```python
from build123d import *

# Parameters (mm, degrees)
SKETCH012_W     = 18.8
SKETCH012_H     = 47
PAD008_DEPTH    = 69
SKETCH036_W     = 14.1
SKETCH036_H     = 47
PAD016_DEPTH    = 2
SKETCH054_R     = 8
POCKET021_DEPTH = 18.801
SKETCH055_R     = 11
POCKET022_DEPTH = 7
CHAMFER001_SIZE = 12
SKETCH073_R     = 1.5
POCKET028_DEPTH = 19.2
FILLET003_R     = 3


with BuildPart() as part:
    # Sketch012 (on Face1 of ReferencePad001) → Pad008 (new body)
    with BuildSketch(Plane.XY.offset(18.8)):
        with Locations((-65.6, 0)):
            Rectangle(SKETCH012_W, SKETCH012_H)
    extrude(amount=PAD008_DEPTH)

    # Sketch036 (on Face5 of Pad008) → Pad016 (join)
    with BuildSketch(Plane(origin=(0, 0, 18.8), x_dir=(1, 0, 0), z_dir=(0, 0, -1))):
        with Locations((-67.95, 0)):
            Rectangle(SKETCH036_W, SKETCH036_H)
    extrude(amount=PAD016_DEPTH)

    # Sketch054 (on Face5 of Pad016) → Pocket021 (cut, through all)
    with BuildSketch(Plane(origin=(-75, 0, 18.8), x_dir=(0, -1, 0), z_dir=(-1, 0, 0))):
        with Locations((0, 56.2)):
            Circle(SKETCH054_R)
    extrude(amount=-POCKET021_DEPTH, mode=Mode.SUBTRACT)

    # Sketch055 (on Face5 of Pocket021) → Pocket022 (cut)
    with BuildSketch(Plane(origin=(-75, 0, 18.8), x_dir=(0, -1, 0), z_dir=(-1, 0, 0))):
        with Locations((0, 56.2)):
            Circle(SKETCH055_R)
    extrude(amount=-POCKET022_DEPTH, mode=Mode.SUBTRACT)

    # Chamfer001
    chamfer001_edges = [part.edges().sort_by_distance(p)[0] for p in [
        (-65.6, -23.5, 87.8),
        (-65.6, 23.5, 87.8),
    ]]
    chamfer(chamfer001_edges, length=CHAMFER001_SIZE)

    # Sketch073 (on Face16 of Chamfer001) → Pocket028 (cut)
    with BuildSketch(Plane(origin=(0, 0, 16.8), x_dir=(1, 0, 0), z_dir=(0, 0, -1))):
        with Locations((-65.6, 11.75)):
            Circle(SKETCH073_R)
        with Locations((-65.6, -11.75)):
            Circle(SKETCH073_R)
    extrude(amount=-POCKET028_DEPTH, mode=Mode.SUBTRACT)

    # Fillet003
    fillet003_edges = [part.edges().sort_by_distance(p)[0] for p in [
        (-65.6, 23.5, 75.8),
        (-65.6, 11.5, 87.8),
        (-65.6, -11.5, 87.8),
        (-65.6, -23.5, 75.8),
    ]]
    fillet(fillet003_edges, radius=FILLET003_R)


solid = part.part
```
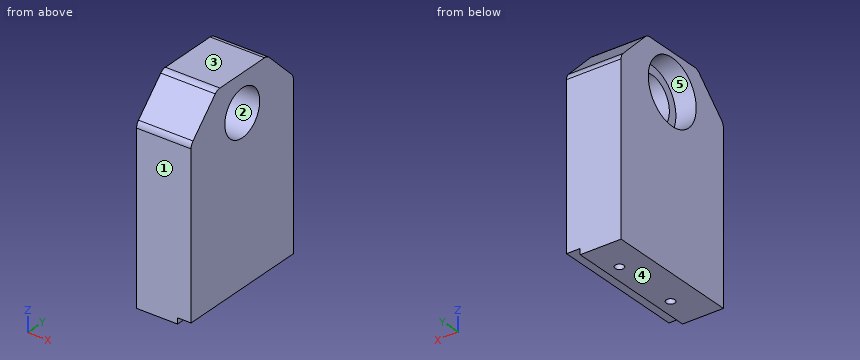
For this review, take the finished solid that the model builds, in its own axes (mm). Face numbers are marked on the shaded views. A direction names the side the tool comes from. Round coordinates to 2 decimals unless told otherwise and drop trailing zeros. Order: outer loops, then holes, each group sorted by start corner. A loop starts at its lowest first (then second) coordinate and runs counter-clockwise, first axis right, second up.
Q1. Insertion check: P1, Ø1.8, axis at x = -65.6, y = 11.75, coming from the -Z side; P2, Ø2.5, axis at x = -58.5, y = -1.5, coming from the -Z side; P3, Ø13, axis at y = 0, z = 75, coming from the -X side; P4, Ø1.6, axis at y = 6.5, z = 17.5, coming from the +X side. Each pin has a flat end and moves straight along its axis. Give the tip position at first contact, or say it passes through.
Findings below:
P1: stops at z = 36
P2: stops at z = 18.8
P3: passes through
P4: stops at x = -60.9
Q2. Machinability: for the marked faces 4 and 5, which of the approach directions +Z, -Z, +X, -X, +Y, -Y give a long, thin tool a straight path to every point of the face, cutting with its end or side? Answer none if there is none.
Findings below:
face 4: -Z, +X, -X, +Y, -Y
face 5: -X
Q3. We need section A-A, the plane x = -65.6. Give the boundary of the cut face in (y, z), plus the area to 3 significant figures.
Findings below:
outline: (-23.5, 16.8) - (-13.25, 16.8) - (-13.25, 36) - (-10.25, 36) - (-10.25, 16.8) - (10.25, 16.8) - (10.25, 36) - (13.25, 36) - (13.25, 16.8) - (23.5, 16.8) - (23.5, 74.56) arc R3 ccw to (22.62, 76.68) - (12.38, 86.92) arc R3 ccw to (10.26, 87.8) - (-10.26, 87.8) arc R3 ccw to (-12.38, 86.92) - (-22.62, 76.68) arc R3 ccw to (-23.5, 74.56) - close; hole circle Ø16 at (0, 75)
area: 2,880 mm2
Q4. Mouldability with a two-part tool opening along Z and no side actions: class the marked faces 1, 2 and 3 as pulls with the +Z half, pulls with the -Z half, needs draft (parallel to the pull), parting line crosses it, or undercut.
Findings below:
face 1: needs draft
face 2: undercut
face 3: pulls with the +Z half
Q5. Wall thickness on line 1 (Y direction, x = -65.6, z = 30.5); line 2 (Z direction, x = -59, y = 0); line 3 (Z direction, x = -71.5, y = 0): over which ranges is each line inside the solid? List them lowest first.
Findings below:
line 1: y = -23.5 to -13.25, -10.25 to 10.25, 13.25 to 23.5
line 2: z = 18.8 to 67, 83 to 87.8
line 3: z = 16.8 to 64, 86 to 87.8
Q6. We need section D-D, the plane x = -69.5. Give the boundary of the cut face in (y, z).
Findings below:
outline: (-23.5, 16.8) - (23.5, 16.8) - (23.5, 74.56) arc R3 ccw to (22.62, 76.68) - (12.38, 86.92) arc R3 ccw to (10.26, 87.8) - (-10.26, 87.8) arc R3 ccw to (-12.38, 86.92) - (-22.62, 76.68) arc R3 ccw to (-23.5, 74.56) - close; hole circle Ø22 at (0, 75)
Q7. We need section C-C, the plane z = 69. Give the boundary of the cut face in (x, y).
Findings below:
outline: (-75, -23.5) - (-56.2, -23.5) - (-56.2, -5.29) - (-68, -5.29) - (-68, -9.22) - (-75, -9.22) - close; (-75, 9.22) - (-68, 9.22) - (-68, 5.29) - (-56.2, 5.29) - (-56.2, 23.5) - (-75, 23.5) - close
Q8. We need section B-B, the plane y = 0. Give the boundary of the cut face in (x, z), plus the area to 3 significant figures.
Findings below:
outline: (-75, 16.8) - (-60.9, 16.8) - (-60.9, 18.8) - (-56.2, 18.8) - (-56.2, 67) - (-68, 67) - (-68, 64) - (-75, 64) - close; (-75, 86) - (-68, 86) - (-68, 83) - (-56.2, 83) - (-56.2, 87.8) - (-75, 87.8) - close
area: 983 mm2
